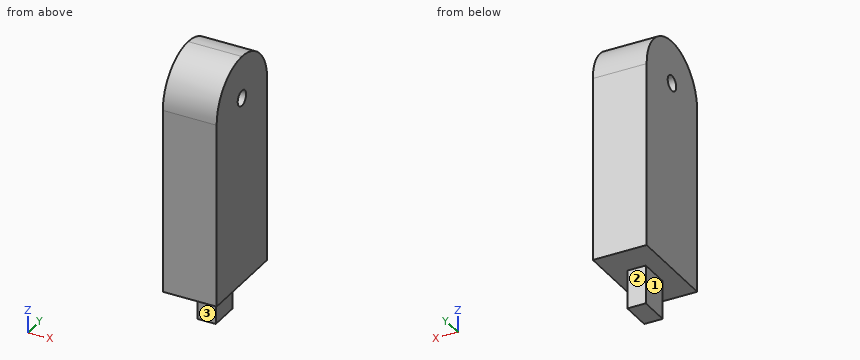
from build123d import *

# Parameters (mm, degrees)
F0_W     = 35
F0_H     = 60
F1_DEPTH = 150
F2_W     = 12
F2_H     = 20
F3_DEPTH = 25
F4_R     = 29.99999
F6_D     = 10


# Not quite as in the source:
# - a fillet or chamfer is up to 0.001 mm smaller than in the source, because OpenCascade refuses the exact size


with BuildPart() as f1:
    # F0 (on Top) → F1 (new body)
    with BuildSketch(Plane.XY):
        Rectangle(F0_W, F0_H)
    extrude(amount=F1_DEPTH)

    # F2 (on face) → F3 (join)
    with BuildSketch(Plane(origin=(0, 0, 0), x_dir=(1, 0, 0), z_dir=(0, 0, -1))):
        Rectangle(F2_W, F2_H)
    extrude(amount=F3_DEPTH)

    # F4 (radius 30 in the source; OpenCascade refuses exactly that, so slightly less here)
    f4_edges = [f1.edges().sort_by_distance(p)[0] for p in [
        (0, -30, 150),
        (0, 30, 150),
    ]]
    fillet(f4_edges, radius=F4_R)

    # F6 (through all)
    with Locations(Plane(origin=(-17.5, 0, 0), x_dir=(0, -1, 0), z_dir=(-1, 0, 0))):
        with Locations((0, 122.46029087)):
            Hole(F6_D / 2)


solid = f1.part
Can you work these out from the model? Positions are in its coordinate system, mm. Face numbers are marked on the shaded views. A direction names the side the tool comes from. Coordinates: 2 decimals unless noted, no trailing zeros. Write each loop counter-clockwise with the first axis right and the second up, starting at its lowest first coordinate (ties: lowest second). Pieces come first, ordered by that corner, then holes.
Q1. Imagine slicing it at D-D, the plane y = -23. List the corners of the cut face in (x, z) for me, plus the area to 3 significant figures.
Results found:
outline: (-17.5, 0) - (17.5, 0) - (17.5, 139.26) - (-17.5, 139.26) - close
area: 4,870 mm2
Q2. Please list where these lines run through material, in increasing order: L1, parallel to Z at x = -1, y = 0; L2, parallel to Z at x = -9, y = -2.5; L3, parallel to Y at x = -0.5, z = 125.
Results found:
L1: z = -25 to 117.46, 127.46 to 150
L2: z = 0 to 118.13, 126.79 to 149.9
L3: y = -29.58 to -4.31, 4.31 to 29.58
Q3. Which directions (+Z, -Z, +X, -X, +Y, -Y) give clear straight access to the entire face, cutting with the end or side of a thin tool? Please do the marked faces 1, 2 and 3.
Results found:
face 1: -Z, -X, +Y, -Y
face 2: -Z, +X, -X, +Y
face 3: -Z, +X, -X, -Y
Q4. For P1, Ø10, axis at y = -4, z = -9, coming from the -X side; P2, Ø9.5, axis at x = 2.5, z = -7.5, coming from the +Y side; P3, Ø5, axis at x = -8, y = 12, coming from the -Z side, each with a flat end and sliding along its axis, tell me the tip position at first contact or that it passes through.
Results found:
P1: stops at x = -6
P2: stops at y = 10
P3: stops at z = 0
Q5. Imagine slicing it at B-B, the plane z = -7. List the corners of the cut face in (x, y) for me, plus the area to 3 significant figures.
Results found:
outline: (-6, -10) - (6, -10) - (6, 10) - (-6, 10) - close
area: 240 mm2
